Input: part model. Units: mm. Frame: model coordinates. A direction names the side the tool comes from. Coordinates: 2 decimals unless noted, no trailing zeros. Order: outer loops, then holes, each group sorted by start corner. A loop starts at its lowest first (then second) coordinate and runs counter-clockwise, first axis right, second up. Notation, with made-up numbers: (-20, -36) - (-15, -36) arc R19 ccw to (-15, -19) - close; hole circle Ø11 at (38, 49.5). An arc over 180 degrees is marked (long way). One line per question, with ' | ' between items. Start each with the question number.
```python
from build123d import *

# Parameters (mm, degrees)
F0_R     = 40
F1_DEPTH = 30
F2_W     = 50
F2_H     = 50
F3_DEPTH = 50
F4_W     = 40
F4_H     = 37.309842


with BuildPart() as f1:
    # F0 (on Top) → F1 (new body)
    with BuildSketch(Plane.XY):
        Circle(F0_R)
    extrude(amount=F1_DEPTH)

    # F2 (on face) → F3 (join)
    with BuildSketch(Plane.XY.offset(30)):
        Rectangle(F2_W, F2_H)
    extrude(amount=F3_DEPTH)

    # F4 (on face) → F6 section 0
    with BuildSketch(Plane.XY.offset(80), mode=Mode.PRIVATE) as f6_s0:
        Rectangle(F4_W, F4_H)
    loft([Vertex(0, 0, 143.321168), f6_s0.sketch])


solid = f1.part
```
(1) Section D-D (z = 94). Output: boundary loops of the cut face in (x, y).
(2) Section C-C (z = 54). Output: boundary loops of the cut face in (x, y), then the cut area to 3 significant figures.
(3) Section A-A (y = -11.5). Output: boundary loops of the cut face in (x, z).
(4) Material intervals for line 1 along X through (y, z) = (-6, 57); line 2 along Z through (x, y) = (-15, -26.5); line 3 along Z through (x, y) = (24, -10.5), sorted ascending. Write a range as from..to.
(5) Reachability of faces 1 (the face through (25, 0, 55)), 2 (the face through (0, -25, 55)), 3 (the face through (-25, 0, 55)), 4 (the face through (0, 25, 55)), 5 (the face through (-23, 0, 80)) from +Z, -Z, +X, -X, +Y, -Y: full face, straight path, thin tool, end or side. Return the list, or none.
(6) Pin query (flat end, axial travel): pin 1 (6 mm diameter, centred on x = -16, z = 25.5, fed in from +Y); pin 2 (3 mm diameter, centred on x = 28.5, y = 9, fed in from +Z); pin 3 (15 mm diameter, centred on x = -5.5, z = 60.5, fed in from -Y). Return the tip coordinate at first contact, or that it passes through.
(7) Section B-B (x = 2). Output: boundary loops of the cut face in (y, z).
Worked answers:
1) outline: (-15.58, -14.53) - (15.58, -14.53) - (15.58, 14.53) - (-15.58, 14.53) - close
2) outline: (-25, -25) - (25, -25) - (25, 25) - (-25, 25) - close | area: 2,500 mm²
3) outline: (-38.31, 0) - (38.31, 0) - (38.31, 30) - (25, 30) - (25, 80) - (20, 80) - (12.33, 104.29) - (-12.33, 104.29) - (-20, 80) - (-25, 80) - (-25, 30) - (-38.31, 30) - close
4) line 1: x = -25..25 | line 2: z = 0..30 | line 3: z = 0..80
5) face 1: +Z, +X, +Y, -Y | face 2: +Z, +X, -X, -Y | face 3: +Z, -X, +Y, -Y | face 4: +Z, +X, -X, +Y | face 5: +Z
6) pin 1: stops at y = 37.83 | pin 2: stops at z = 30 | pin 3: stops at y = -25
7) outline: (-39.95, 0) - (39.95, 0) - (39.95, 30) - (25, 30) - (25, 80) - (18.65, 80) - (1.87, 136.99) - (-1.87, 136.99) - (-18.65, 80) - (-25, 80) - (-25, 30) - (-39.95, 30) - close
